```python
from build123d import *

# Parameters (mm, degrees)
BOSS_EXTRUDE2_DEPTH = 48.5
BOSS_EXTRUDE3_DEPTH = 18
SKETCH3_R           = 1.6
CUT_EXTRUDE1_DEPTH  = 8
CUT_EXTRUDE3_DEPTH  = 3
SKETCH5_W           = 78.5
SKETCH5_H           = 16
BOSS_EXTRUDE4_DEPTH = 2
BOSS_EXTRUDE5_DEPTH = 7
BOSS_EXTRUDE6_DEPTH = 7
SKETCH10_R          = 2.1
CUT_EXTRUDE4_DEPTH  = 17
CUT_EXTRUDE5_DEPTH  = 3
CUT_EXTRUDE6_DEPTH  = 79.5


with BuildPart() as part:
    # Sketch1 → Boss-Extrude2 (new body)
    with BuildSketch(Plane.XY):
        Polygon((0.472150472, 5.388924764), (0.472150472, 8.388924764), (-17.527849528, 8.388924764), (-17.527849528, -7.611075236), (0.472150472, -7.611075236), (0.472150472, -4.611075236), align=None)
    extrude(amount=BOSS_EXTRUDE2_DEPTH)

    # Sketch2 → Boss-Extrude3 (add)
    with BuildSketch(Plane.ZY.offset(17.527849528)):
        Polygon((48.5, 8.388924764), (62.5, 8.388924764), (63.5, 8.388924764), (63.5, 7.388924764), (63.5, -6.611075236), (63.5, -7.611075236), (62.5, -7.611075236), (48.5, -7.611075236), (48.5, -4.811075236), (48.5, 5.588924764), align=None)
        Polygon((0, -4.811075236), (0, -7.611075236), (-14, -7.611075236), (-15, -7.611075236), (-15, -6.611075236), (-15, 7.388924764), (-15, 8.388924764), (-14, 8.388924764), (0, 8.388924764), (0, 5.588924764), align=None)
    extrude(amount=-BOSS_EXTRUDE3_DEPTH)

    # Sketch3 → Cut-Extrude1 (cut)
    with BuildSketch(Plane.XY.offset(63.5)):
        with Locations((-9.527849528, 0.388924764)):
            Circle(SKETCH3_R)
    cut_extrude1 = extrude(amount=-CUT_EXTRUDE1_DEPTH, mode=Mode.SUBTRACT)

    # Mirror1: Cut-Extrude1 across plane
    add(cut_extrude1.mirror(Plane.XY.offset(24.25)), mode=Mode.SUBTRACT)

    # Sketch4 → Cut-Extrude3 (cut)
    with BuildSketch(Plane.XY.offset(63.5)):
        Polygon((-7.807950928, -2.618058576), (-6.063776267, 0.374908974), (-7.783674867, 3.381892314), (-11.247748128, 3.395908104), (-12.991922789, 0.402940554), (-11.272024189, -2.604042786), align=None)
    cut_extrude3 = extrude(amount=-CUT_EXTRUDE3_DEPTH, mode=Mode.SUBTRACT)

    # Mirror2: Cut-Extrude3 across plane
    add(cut_extrude3.mirror(Plane.XY.offset(24.25)), mode=Mode.SUBTRACT)

    # Sketch5 → Boss-Extrude4 (add)
    with BuildSketch(Plane.ZY.offset(17.527849528)):
        with Locations((24.25, 0.388924764)):
            Rectangle(SKETCH5_W, SKETCH5_H)
    extrude(amount=BOSS_EXTRUDE4_DEPTH)

    # Sketch6 → Boss-Extrude5 (add)
    with BuildSketch(Plane.XY.offset(63.5)):
        with BuildLine():
            Line((-19.527849528, -7.611075236), (-19.527849528, -8.257098609))
            ThreePointArc((-19.527849528, -8.257098609), (-29.816107458, -10.948302934), (-39.527849528, -15.28107317))
            Line((-39.527849528, -15.28107317), (-39.527849528, -18.149551009))
            ThreePointArc((-39.527849528, -18.149551009), (-8.277849528, -9.776138745), (22.972150472, -18.149551009))
            Line((22.972150472, -18.149551009), (22.972150472, -15.28107317))
            ThreePointArc((22.972150472, -15.28107317), (12.062731895, -10.540729559), (0.472150472, -7.867773606))
            Line((0.472150472, -7.867773606), (0.472150472, -7.611075236))
            Line((0.472150472, -7.611075236), (-19.527849528, -7.611075236))
        make_face()
    boss_extrude5 = extrude(amount=-BOSS_EXTRUDE5_DEPTH)

    # Mirror3: Boss-Extrude5 across plane
    add(boss_extrude5.mirror(Plane.XY.offset(24.25)))

    # Sketch7 → Boss-Extrude6 (add)
    with BuildSketch(Plane.XY.offset(63.5)):
        with BuildLine():
            Line((22.972150472, -18.149551009), (22.972150472, -15.28107317))
            ThreePointArc((22.972150472, -15.28107317), (28.129444831, -18.429050454), (32.972150472, -22.042310502))
            Line((32.972150472, -22.042310502), (32.972150472, -25.322038818))
            ThreePointArc((32.972150472, -25.322038818), (28.149113636, -21.489069971), (22.972150472, -18.149551009))
        make_face()
        with BuildLine():
            Line((-39.527849528, -15.28107317), (-39.527849528, -18.149551009))
            ThreePointArc((-39.527849528, -18.149551009), (-44.704812692, -21.489069971), (-49.527849528, -25.322038818))
            Line((-49.527849528, -25.322038818), (-49.527849528, -22.042310502))
            ThreePointArc((-49.527849528, -22.042310502), (-44.685143887, -18.429050454), (-39.527849528, -15.28107317))
        make_face()
    boss_extrude6 = extrude(amount=-BOSS_EXTRUDE6_DEPTH)

    # Mirror4: Boss-Extrude6 across plane
    add(boss_extrude6.mirror(Plane.XY.offset(24.25)))

    # Sketch10 → Cut-Extrude4 (cut, through all)
    with BuildSketch(Plane.XZ.offset(7.611075236)):
        with Locations((-9.527849528, 40.375)):
            Circle(SKETCH10_R)
        with Locations((-9.527849528, 8.125)):
            Circle(SKETCH10_R)
        with Locations((-9.527849528, 24.25)):
            Circle(SKETCH10_R)
    extrude(amount=-CUT_EXTRUDE4_DEPTH, mode=Mode.SUBTRACT)

    # Sketch11 → Cut-Extrude5 (cut)
    with BuildSketch(Plane(origin=(0, 8.388924764, 0), x_dir=(1, 0, 0), z_dir=(0, 1, 0))):
        Polygon((-7.780505993, -11.116118615), (-6.063793054, -8.107315417), (-7.811136589, -5.116196802), (-11.275193063, -5.133881385), (-12.991906002, -8.142684583), (-11.244562467, -11.133803198), align=None)
        Polygon((-11.244562467, -37.366196802), (-7.780505993, -37.383881385), (-6.063793054, -40.392684583), (-7.811136589, -43.383803198), (-11.275193063, -43.366118615), (-12.991906002, -40.357315417), align=None)
        Polygon((-6.063747913, -24.25), (-7.79579872, -21.25), (-11.259900336, -21.25), (-12.991951143, -24.25), (-11.259900336, -27.25), (-7.79579872, -27.25), align=None)
    extrude(amount=-CUT_EXTRUDE5_DEPTH, mode=Mode.SUBTRACT)

    # Sketch12 → Cut-Extrude6 (cut, through all)
    with BuildSketch(Plane.XY.offset(63.5)):
        with BuildLine():
            Line((5.472150472, -8.747109948), (5.472150472, -11.307396754))
            ThreePointArc((5.472150472, -11.307396754), (20.100884553, -16.590436344), (32.972150472, -25.322038818))
            Line((32.972150472, -25.322038818), (32.972150472, -22.042310502))
            ThreePointArc((32.972150472, -22.042310502), (20.014209242, -13.756403523), (5.472150472, -8.747109948))
        make_face()
    extrude(amount=-CUT_EXTRUDE6_DEPTH, mode=Mode.SUBTRACT)


solid = part.part
```
Geometry: final body of the model. Coordinates: model frame, mm. A direction names the side the tool comes from. Round coordinates to 2 decimals unless told otherwise and drop trailing zeros. Order: outer loops, then holes, each group sorted by start corner. A loop starts at its lowest first (then second) coordinate and runs counter-clockwise, first axis right, second up. Notation, with made-up numbers: (80, 71) - (94, 71) arc R28 cw to (94, 98) - close; hole circle Ø9 at (89.5, -12.75). An arc over 180 degrees is marked (long way). Write item = value, one per line. Start each with the question number.
Q1. Pin query (flat end, axial travel): pin 1 (5.5 mm diameter, centred on x = -9.53, z = 24.25, fed in from -Y); pin 2 (3 mm diameter, centred on x = -9.5, z = 8, fed in from +Y); pin 3 (4 mm diameter, centred on y = -2, z = 27.5, fed in from +X); pin 4 (6.5 mm diameter, centred on x = -9.53, z = 40.38, fed in from +Y). Return the tip coordinate at first contact, or that it passes through.
Q2. Cut plane B-B on y = -16.5. Return the cut outline in (x, z), and give its area (3 significant figures).
Q3. Cut plane A-A on x = -30.5. Return the cut outline in (y, z), and give its area (3 significant figures).
Q4. Cut plane C-C on y = -6. Return the cut outline in (x, z) (3 decimals), and give its area (3 significant figures).
Q5. Ray query, line 1 (Z direction, x = -30.5, y = -12); line 2 (Z direction, x = -11, y = 6.5); line 3 (Z direction, x = -8, y = -6). Return the intervals inside material, ascending. Write a range as from..to.
Q6. Pull-direction query (Z, two-part tool) for faces 1 (the flat face through (-10, 0, -7)), 2 (the flat face through (0.472, 0, 24)), 3 (the flat face through (-12.13, 6.91, 9.62)); classes: +Z half, -Z half, draft (parallel to the pull), parting line (faces both ways), or undercut.
Q7. Access query for faces 4 (the flat face through (-24, -11, 56.5)), 5 (the flat face through (-19.528, 0, 24)), 6 (the flat face through (-12.122, 6.91, 41.883)), 7 (the cylindrical face through (-9.875, -1.173, 58.035)). Directions: +Z, -Z, +X, -X, +Y, -Y. A direction counts if a zero-diameter tool reaches every point of the face in a straight line with its end or side. Return the directions, or none.
Q8. Cut plane D-D on x = -10. Give the number of separate pieces and of enclosed holes in the cut face, and give its area (3 significant figures).
Outcome:
q1.pin_1 = -7.61
q1.pin_2 = through
q1.pin_3 = 0.47
q1.pin_4 = 8.39
q2.outline = (-41.65, -15) - (-36.48, -15) - (-36.48, -8) - (-41.65, -8) - close; (-41.65, 56.5) - (-36.48, 56.5) - (-36.48, 63.5) - (-41.65, 63.5) - close
q2.area = 72.5 mm^2
q3.outline = (-13.86, -15) - (-11.19, -15) - (-11.19, -8) - (-13.86, -8) - close; (-13.86, 56.5) - (-11.19, 56.5) - (-11.19, 63.5) - (-13.86, 63.5) - close
q3.area = 37.3 mm^2
q4.outline = (-19.528, -15) - (0.472, -15) - (0.472, 63.5) - (-19.528, 63.5) - close; hole circle Ø4.2 at (-9.528, 8.125); hole circle Ø4.2 at (-9.528, 24.25); hole circle Ø4.2 at (-9.528, 40.375)
q4.area = 1,530 mm^2
q5.line_1 = -15..-8, 56.5..63.5
q5.line_2 = -15..5.13, 11.13..21.25, 27.25..37.37, 43.37..63.5
q5.line_3 = -15..6.68, 9.57..22.81, 25.69..38.93, 41.82..63.5
q6.face_1 = -Z half
q6.face_2 = draft
q6.face_3 = undercut
q7.face_4 = +X, -X, -Y
q7.face_5 = +Z, -Z, -X, +Y
q7.face_6 = +Y
q7.face_7 = +Z
q8.separate_pieces = 4
q8.enclosed_holes = 0
q8.area = 1,010 mm^2
